Check sheet for the drawn part. Datum: minimum x, y, z corner. Units: mm. A direction names the side the tool comes from. Round coordinates to 2 decimals unless told otherwise and drop trailing zeros. Write each loop counter-clockwise with the first axis right and the second up, starting at its lowest first coordinate (ties: lowest second). Pieces come first, ordered by that corner, then holes. Notation, with made-up numbers: M -8.75,39 L 40.25,39 A22 ccw 40.25,53 Z; hole C -34,-30 d6. An arc over 180 degrees is marked long. Use a Markdown table: item, result.
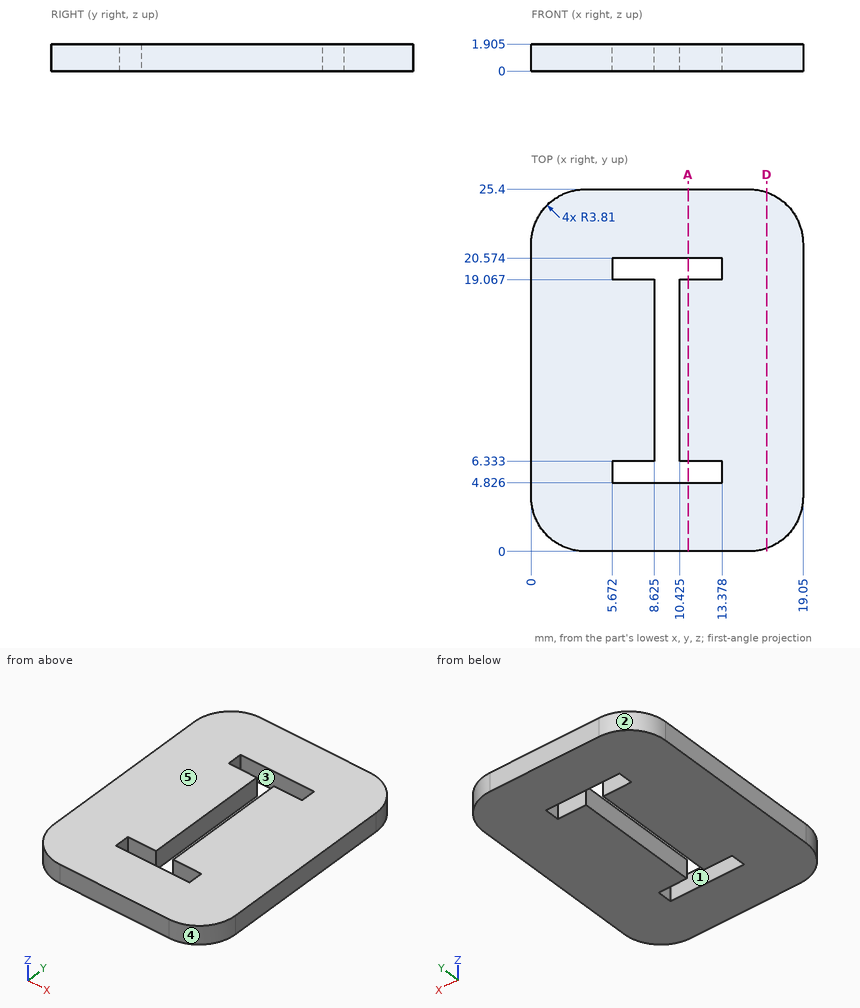
Item 1: Material ranges on line 1 along Y through (x, z) = (13, 1.4); line 2 along Y through (x, z) = (10, 1.1); line 3 along X through (y, z) = (22.5, 0.45), recorded low to high. Write a range as from..to.
Outcome:
| item | result |
|---|---|
| line 1 | y = 0..4.83, 6.33..19.07, 20.57..25.4 |
| line 2 | y = 0..4.83, 20.57..25.4 |
| line 3 | x = 0.11..18.94 |
Item 2: Access from +Z, -Z, +X, -X, +Y, -Y to the whole of each face (thin tool, end or side, straight path). Record for the marked faces 1 and 2.
Outcome:
| item | result |
|---|---|
| face 1 | +Z, -Z |
| face 2 | +Z, -Z, -X, +Y |
Item 3: Cross-section at A-A, the plane x = 11. Record the cut outline in (y, z) (1 decimal).
Outcome:
| item | result |
|---|---|
| outline | M 0,0 L 4.8,0 L 4.8,1.9 L 0,1.9 Z; M 6.3,0 L 19.1,0 L 19.1,1.9 L 6.3,1.9 Z; M 20.6,0 L 25.4,0 L 25.4,1.9 L 20.6,1.9 Z |
Item 4: Mould release check, pull along X, two halves, no side actions. Record for the marked faces 3, 4 and 5: +X half, -X half, draft (parallel to the pull), parting line (faces both ways), or undercut.
Outcome:
| item | result |
|---|---|
| face 3 | undercut |
| face 4 | +X half |
| face 5 | draft |
Item 5: Cross-section at D-D, the plane x = 16.5. Record the cut outline in (y, z) (1 decimal).
Outcome:
| item | result |
|---|---|
| outline | M 0.2,0 L 25.2,0 L 25.2,1.9 L 0.2,1.9 Z |
